Autodesk Inventor part; units mm, degrees
ref_plane "YZ Plane" through (0, 0, 0) normal (1, 0, 0) x (0, 1, 0)
ref_plane "XZ Plane" through (0, 0, 0) normal (0, 1, 0) x (-1, 0, 0)
ref_plane "XY Plane" through (0, 0, 0) normal (0, 0, 1) x (1, 0, 0)
sketch "Sketch1" plane through (0, 0, 0) normal (0, 1, 0) x (-1, 0, 0)
  line L0 (0, 0) -> (15, 0)
  line L1 (15, 0) -> (15, -10)
  line L2 (15, -10) -> (0, -10)
  line L3 (0, -10) -> (0, 0)
  dimension "d0" = 15
  dimension "d1" = 10
extrude "Extrusion1" add sketch "Sketch1" along normal blind 10
sketch "Sketch2" plane through (-15, 0, 0) normal (0, 0, 1) x (1, 0, 0)
  line L0 (15, 0) -> (0, 0)
  line L1 (15, 0) -> (15, 10)
  line L2 (0, 0) -> (15, 0)
  line L3 (15, 0) -> (15, 2.75)
  line L4 (15, 2.75) -> (0, 2.75)
  line L5 (0, 2.75) -> (0, 0)
  dimension "d4" = 2.75
extrude "Extrusion2" cut sketch "Sketch2" against normal blind 2.75
sketch "Sketch3" plane through (0, 0, -10) normal (1, 0, 0) x (0, 0, -1)
  line L0 (0, 10) -> (-2.75, 10)
  line L1 (-2.75, 10) -> (-2.75, 7.25)
  line L2 (-2.75, 7.25) -> (0, 7.25)
  line L3 (0, 7.25) -> (0, 10)
  point P0 (-10, 0)
  dimension "d7" = 2.75
  dimension "d8" = 2.75
extrude "Extrusion3" cut sketch "Sketch3" against normal blind 15
sketch "Sketch4" plane through (0, 10, 0) normal (0, 1, 0) x (1, 0, 0)
  line L0 (0, 7.25) -> (-15, 7.25)
  line L1 (-10, 7.25) -> (-4, 7.25)
  line L2 (-4, 7.25) -> (-4, 4.5)
  line L3 (-4, 4.5) -> (-10, 4.5)
  line L4 (-10, 4.5) -> (-10, 7.25)
  dimension "d11" = 6
  dimension "d12" = 2.75
extrude "Extrusion4" cut sketch "Sketch4" against normal blind 2.75
sketch "Sketch5" plane through (0, 0, -2.75) normal (1, 0, 0) x (0, 0, -1)
  line L0 (0, 4.5) -> (4.5, 4.5)
  line L1 (4.5, 4.5) -> (4.5, 5.5)
  line L2 (4.5, 5.5) -> (0, 5.5)
  line L3 (0, 5.5) -> (0, 4.5)
  point P0 (-2.75, 0)
  dimension "d15" = 1
extrude "Extrusion5" cut sketch "Sketch5" against normal blind 15
properties part number "148"
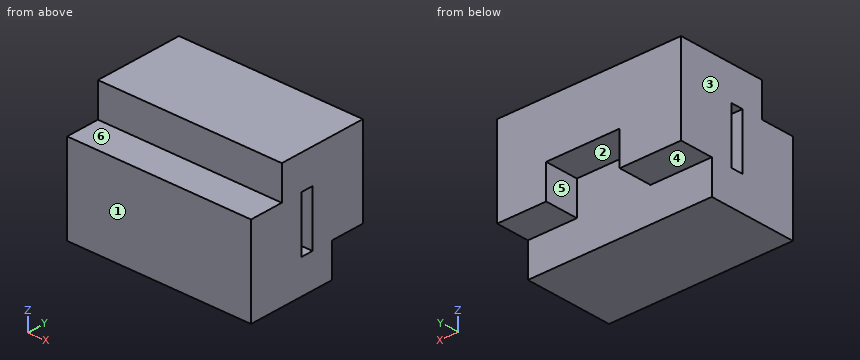
Design review of the part built by this model. Coordinates are the model's own, in mm. Face numbers are marked on the shaded views. A direction names the side the tool comes from. Coordinates: 2 decimals unless noted, no trailing zeros. Order: outer loops, then holes, each group sorted by start corner. A loop starts at its lowest first (then second) coordinate and runs counter-clockwise, first axis right, second up. Notation, with made-up numbers: M -4.75,-39.75 L 29.25,-39.75 A26 ccw 29.25,-16.75 Z; hole C 38.5,80.5 d10. An arc over 180 degrees is marked long. Answer as a JSON object with one key per item and string values. Group by question number.
1) Wall thickness on L1, parallel to Y at x = -12.25, z = -7; L2, parallel to Z at x = -12.5, y = 5; L3, parallel to Y at x = -9, z = -0.5: over which ranges is each line inside the solid? List them lowest first.
2) Add section B-B, the plane z = -5.75. Write out the cut boundary in (x, y).
3) Tool access review of the marked faces 4, 5 and 6: name each direction out of +Z, -Z, +X, -X, +Y, -Y from which nothing blocks a thin tool from reaching the whole face with its end or side.
4) Add section C-C, the plane y = 8.5. Write out the cut boundary in (x, z).
5) Add section A-A, the plane x = -8.25. Write out the cut boundary in (y, z), then the cut area to 3 significant figures.
6) Mouldability with a two-part tool opening along X and no side actions: class the marked faces 1, 2 and 3 as pulls with the +X half, pulls with the -X half, needs draft (parallel to the pull), parting line crosses it, or undercut.
7) Add section D-D, the plane x = -3.5. Write out the cut boundary in (y, z), then the cut area to 3 significant figures.
8) For pin 1 (2 mm diameter, centred on x = -11, z = -1, fed in from -Y); pin 2 (3 mm diameter, centred on x = -7, y = 9, fed in from -Z); pin 3 (3 mm diameter, centred on x = -3, y = 9, fed in from -Z), all flat-tipped, find the tip position at first contact; note any pin that passes through.
Computed values:
{
 "1": {"L1": "y = 0 to 4.5, 5.5 to 10", "L2": "z = -10 to -7.25, -2.75 to 0", "L3": "y = 2.75 to 10"},
 "2": {"outline": "M -15,0 L 0,0 L 0,4.5 L -15,4.5 Z; M -15,5.5 L 0,5.5 L 0,10 L -4,10 L -4,7.25 L -10,7.25 L -10,10 L -15,10 Z"},
 "3": {"face 4": "-Z, +X, -X, +Y", "face 5": "-Z, +Y", "face 6": "+Z, +X, -X, -Y"},
 "4": {"outline": "M -15,-7.25 L -10,-7.25 L -10,-4.5 L -4,-4.5 L -4,-7.25 L 0,-7.25 L 0,0 L -15,0 Z"},
 "5": {"outline": "M 0,-10 L 7.25,-10 L 7.25,-4.5 L 10,-4.5 L 10,0 L 2.75,0 L 2.75,-2.75 L 0,-2.75 Z; hole M 4.5,-7.25 L 5.5,-7.25 L 5.5,-2.75 L 4.5,-2.75 Z", "area": "72.8 mm^2"},
 "6": {"face 1": "needs draft", "face 2": "undercut", "face 3": "pulls with the -X half"},
 "7": {"outline": "M 0,-10 L 7.25,-10 L 7.25,-7.25 L 10,-7.25 L 10,0 L 2.75,0 L 2.75,-2.75 L 0,-2.75 Z; hole M 4.5,-7.25 L 5.5,-7.25 L 5.5,-2.75 L 4.5,-2.75 Z", "area": "80.4 mm^2"},
 "8": {"pin 1": "stops at y = 2.75", "pin 2": "stops at z = -4.5", "pin 3": "stops at z = -7.25"}
}
